from build123d import *

# Parameters (mm, degrees)
SKETCH6_W           = 72
SKETCH6_H           = 25
BOSS_EXTRUDE2_DEPTH = 46
SKETCH9_R           = 1.6
CUT_EXTRUDE3_DEPTH  = 35
TOP_SCREW_HOLES_D   = 5
SKETCH12_W          = 36
SKETCH12_H          = 24
CUT_EXTRUDE4_DEPTH  = 64.537390567
SKETCH13_W          = 30
SKETCH13_H          = 25
CUT_EXTRUDE5_DEPTH  = 17
CUT_EXTRUDE6_START  = 25
SKETCH14_R          = 16.5
CUT_EXTRUDE6_DEPTH  = 16


with BuildPart() as part:
    # Sketch6 → Boss-Extrude2 (new body)
    with BuildSketch(Plane(origin=(0, 0, 0), x_dir=(1, 0, 0), z_dir=(0, 1, 0))):
        Rectangle(SKETCH6_W, SKETCH6_H)
    extrude(amount=BOSS_EXTRUDE2_DEPTH)

    # Sketch9 → Cut-Extrude3 (cut)
    with BuildSketch(Plane(origin=(0, 46, 0), x_dir=(1, 0, 0), z_dir=(0, 1, 0))):
        with Locations(Location((-33, 9.3, 0), (0, 0, 270))):
            Circle(SKETCH9_R)
        with Locations(Location((33, 9.3, 0), (0, 0, 90))):
            Circle(SKETCH9_R)
    extrude(amount=-CUT_EXTRUDE3_DEPTH, mode=Mode.SUBTRACT)

    # Top Screw Holes (through all)
    with Locations(Plane(origin=(0, 46, 0), x_dir=(1, 0, 0), z_dir=(0, 1, 0))):
        with Locations((-22.5, -7.5), (22.5, -7.5), (-22.5, 7.5), (22.5, 7.5)):
            Hole(TOP_SCREW_HOLES_D / 2)

    # Sketch12 → Cut-Extrude4 (cut, through all)
    with BuildSketch(Plane.XY.offset(12.5)):
        with Locations((0, 12)):
            Rectangle(SKETCH12_W, SKETCH12_H)
    extrude(amount=-CUT_EXTRUDE4_DEPTH, mode=Mode.SUBTRACT)

    # Sketch13 → Cut-Extrude5 (cut)
    with BuildSketch(Plane(origin=(0, 46, 0), x_dir=(1, 0, 0), z_dir=(0, 1, 0))):
        Rectangle(SKETCH13_W, SKETCH13_H)
    extrude(amount=-CUT_EXTRUDE5_DEPTH, mode=Mode.SUBTRACT)

    # Sketch14 → Cut-Extrude6 (cut)
    with BuildSketch(Plane(origin=(0, 0, 0), x_dir=(1, 0, 0), z_dir=(0, 1, 0)).offset(CUT_EXTRUDE6_START)):
        with Locations((-33, 9.3)):
            Circle(SKETCH14_R)
        with Locations((33, 9.3)):
            Circle(SKETCH14_R)
    extrude(amount=CUT_EXTRUDE6_DEPTH, mode=Mode.SUBTRACT)


solid = part.part
Read the model definition and answer for the solid it produces. Units are mm, in the model's axes. A direction names the side the tool comes from. Give positions to 0.01 mm unless a question says otherwise; leave off trailing zeros. Loops run counter-clockwise (first coordinate to the right, second up) from the corner with the lowest first, then second, coordinate; pieces in that order, holes last. Notation, with made-up numbers: (63, 55.25) - (105, 55.25) arc R26 ccw to (105, 90.25) - close; hole circle Ø8 at (62.5, 8.25). An arc over 180 degrees is marked (long way). Answer as CSV lines item,"result". Start each with the question number.
1) Find section C-C (y = 22.5). Write down the section's boundary in (x, z).
2) Straight lines are drawn through the part: L1, parallel to Z at x = -22.5, y = 43.8; L2, parallel to X at y = 13.5, z = -11; L3, parallel to Z at x = 22, y = 21. For each, find the intervals that lie inside material, in ascending order. Write a range as from..to.
3) Find section A-A (y = 7.5). Write down the section's boundary in (x, z).
4) Find section B-B (x = -33). Write down the section's boundary in (y, z).
5) Which of the six approach directions +Z, -Z, +X, -X, +Y, -Y give full straight-line access (tool end or side, diameter ignored) to faces 1 (the face through (-18, 12, 0)), 2 (the face through (24.5, 22.7, 9)), 3 (the face through (33, 11, -9)), 4 (the face through (21.1, 32.89, 2.13)), 5 (the face through (-15, 38, 0))?
6) Find section D-D (x = 21). Write down the section's boundary in (y, z).
7) Each of these flat-tipped pins is pushed along its axis until it touches: pin 1 Ø10 at (x, z) = (5, 6) entering from -Y; pin 2 Ø1.6 at (x, z) = (-33.5, -9) entering from +Y; pin 3 Ø6 at (y, z) = (31, 1.5) entering from -X. Where does it stop, or does it pass through?
8) Determine the mould class of faces 6 (the face through (18, 12, 0)), 7 (the face through (-36, 18, 0)), 8 (the face through (-27, 0, 0)) for opening direction X: released by +X, released by -X, zero draft, split by the parting line, or undercut.
Findings below:
1,outline,"(-36, -12.5) - (-18, -12.5) - (-18, 12.5) - (-36, 12.5) - close; (18, -12.5) - (36, -12.5) - (36, 12.5) - (18, 12.5) - close; hole circle Ø3.2 at (-33, -9.3); hole circle Ø5 at (-22.5, -7.5); hole circle Ø5 at (-22.5, 7.5); hole circle Ø5 at (22.5, -7.5); hole circle Ø5 at (22.5, 7.5); hole circle Ø3.2 at (33, -9.3)"
2,L1,"-12.5..-10, -5..5, 10..12.5"
2,L2,"-36..-18, 18..36"
2,L3,"-12.5..-9.95, -5.05..5.05, 9.95..12.5"
3,outline,"(-36, -12.5) - (-18, -12.5) - (-18, 12.5) - (-36, 12.5) - close; (18, -12.5) - (36, -12.5) - (36, 12.5) - (18, 12.5) - close; hole circle Ø5 at (-22.5, -7.5); hole circle Ø5 at (-22.5, 7.5); hole circle Ø5 at (22.5, -7.5); hole circle Ø5 at (22.5, 7.5)"
4,outline,"(0, -12.5) - (25, -12.5) - (25, -10.9) - (11, -10.9) - (11, -7.7) - (25, -7.7) - (25, 7.2) - (41, 7.2) - (41, -7.7) - (46, -7.7) - (46, 12.5) - (0, 12.5) - close; (41, -12.5) - (46, -12.5) - (46, -10.9) - (41, -10.9) - close"
5,face 1,"+Z, -Z, -Y"
5,face 2,"+Y, -Y"
5,face 3,"+Y"
5,face 4,"none"
5,face 5,"+Z, -Z, +Y"
6,outline,"(0, -12.5) - (25, -12.5) - (25, -9.5) - (0, -9.5) - close; (0, -5.5) - (25, -5.5) - (25, 2.02) - (41, 2.02) - (41, -5.5) - (46, -5.5) - (46, 5.5) - (0, 5.5) - close; (0, 9.5) - (46, 9.5) - (46, 12.5) - (0, 12.5) - close; (41, -12.5) - (46, -12.5) - (46, -9.5) - (41, -9.5) - close"
7,pin 1,"y = 24"
7,pin 2,"y = 11"
7,pin 3,"x = -23.96"
8,face 6,"undercut"
8,face 7,"released by -X"
8,face 8,"zero draft"
